```python
from build123d import *

# Parameters (mm, degrees)
BOSS_EXTRUDE1_DEPTH = 20
SKETCH2_R           = 4.835
BOSS_EXTRUDE2_DEPTH = 4
CUT_EXTRUDE1_REACH  = 64.738
SKETCH3_R           = 7.665
CUT_EXTRUDE2_DEPTH  = 10
SKETCH5_W           = 6
SKETCH5_H           = 4
CUT_EXTRUDE3_DEPTH  = 10
CUT_EXTRUDE4_REACH  = 64.738
SKETCH6_R           = 1.165


with BuildPart() as part:
    # Sketch1 → Boss-Extrude1 (new body)
    with BuildSketch(Plane.XY):
        Polygon((-40.25, -10), (-40.25, -6), (-50, -6), (-56, -6), (-56, 6), (-50, 6), (-40.25, 6), (-40.25, 10), (0, 10), (2.25, 10), (2.25, 6), (0, 6), (-9.75, 6), (-9.75, -6), (0, -6), (2.25, -6), (2.25, -10), (0, -10), align=None)
    extrude(amount=BOSS_EXTRUDE1_DEPTH)

    # Sketch2 → Boss-Extrude2 (add)
    with BuildSketch(Plane.XZ.offset(6)):
        with Locations(Location((-50, 10, 0), (0, 0, 180))):
            Circle(SKETCH2_R)
    boss_extrude2 = extrude(amount=BOSS_EXTRUDE2_DEPTH)

    # Cut-Extrude1: up to this face of the body (flat: up to its plane)
    cut_extrude1_end = Plane(part.part.faces().sort_by_distance((-19, 10, 10))[0])
    # Sketch3 → Cut-Extrude1 (cut, up to the picked face)
    with BuildSketch(Plane.XZ.offset(10), mode=Mode.PRIVATE) as cut_extrude1_sk1:
        with Locations((0, 10)):
            Circle(SKETCH3_R)
    cut_extrude1_tool1 = split(extrude(cut_extrude1_sk1.sketch, amount=-CUT_EXTRUDE1_REACH, mode=Mode.PRIVATE), bisect_by=cut_extrude1_end, keep=Keep.BOTH, mode=Mode.PRIVATE)
    add(cut_extrude1_tool1.solids().sort_by(Axis((0, -10, 10), (0, 1, 0)))[0], mode=Mode.SUBTRACT)

    # Mirror1: Boss-Extrude2 across plane
    add(boss_extrude2.mirror(Plane.ZX))

    # Sketch4 → Cut-Extrude2 (cut)
    with BuildSketch(Plane.XY.offset(20)):
        Polygon((-27.5, 2.5), (-22.5, 2.062556682), (-22.5, -2.062556682), (-27.5, -2.5), align=None)
    extrude(amount=-CUT_EXTRUDE2_DEPTH, mode=Mode.SUBTRACT)

    # Sketch5 → Cut-Extrude3 (cut)
    with BuildSketch(Plane.XY.offset(20)):
        with Locations((-30.5, 5.165)):
            Rectangle(SKETCH5_W, SKETCH5_H)
        with Locations((-19.5, 5.165)):
            Rectangle(SKETCH5_W, SKETCH5_H)
        with Locations((-19.5, -5.165)):
            Rectangle(SKETCH5_W, SKETCH5_H)
        with Locations((-30.5, -5.165)):
            Rectangle(SKETCH5_W, SKETCH5_H)
    extrude(amount=-CUT_EXTRUDE3_DEPTH, mode=Mode.SUBTRACT)

    # Cut-Extrude4: up to this face of the body (flat: up to its plane)
    cut_extrude4_end = Plane(part.part.faces().sort_by_distance((-21.952820108, 10, 10))[0])
    # Sketch6 → Cut-Extrude4 (cut, up to the picked face)
    with BuildSketch(Plane.XZ.offset(10), mode=Mode.PRIVATE) as cut_extrude4_sk1:
        with Locations(Location((-30.5, 13, 0), (0, 0, 270))):
            Circle(SKETCH6_R)
    cut_extrude4_tool1 = split(extrude(cut_extrude4_sk1.sketch, amount=-CUT_EXTRUDE4_REACH, mode=Mode.PRIVATE), bisect_by=cut_extrude4_end, keep=Keep.BOTH, mode=Mode.PRIVATE)
    # Sketch6 → Cut-Extrude4 (cut, up to the picked face)
    with BuildSketch(Plane.XZ.offset(10), mode=Mode.PRIVATE) as cut_extrude4_sk2:
        with Locations((-25, 13)):
            Circle(SKETCH6_R)
    cut_extrude4_tool2 = split(extrude(cut_extrude4_sk2.sketch, amount=-CUT_EXTRUDE4_REACH, mode=Mode.PRIVATE), bisect_by=cut_extrude4_end, keep=Keep.BOTH, mode=Mode.PRIVATE)
    # Sketch6 → Cut-Extrude4 (cut, up to the picked face)
    with BuildSketch(Plane.XZ.offset(10), mode=Mode.PRIVATE) as cut_extrude4_sk3:
        with Locations(Location((-19.5, 13, 0), (0, 0, 90))):
            Circle(SKETCH6_R)
    cut_extrude4_tool3 = split(extrude(cut_extrude4_sk3.sketch, amount=-CUT_EXTRUDE4_REACH, mode=Mode.PRIVATE), bisect_by=cut_extrude4_end, keep=Keep.BOTH, mode=Mode.PRIVATE)
    add(cut_extrude4_tool1.solids().sort_by(Axis((-30.5, -10, 13), (0, 1, 0)))[0], mode=Mode.SUBTRACT)
    add(cut_extrude4_tool2.solids().sort_by(Axis((-25, -10, 13), (0, 1, 0)))[0], mode=Mode.SUBTRACT)
    add(cut_extrude4_tool3.solids().sort_by(Axis((-19.5, -10, 13), (0, 1, 0)))[0], mode=Mode.SUBTRACT)


solid = part.part
```
Geometry: final body of the model. Coordinates: model frame, mm. A direction names the side the tool comes from. Give positions to 0.01 mm unless a question says otherwise; leave off trailing zeros. Order: outer loops, then holes, each group sorted by start corner. A loop starts at its lowest first (then second) coordinate and runs counter-clockwise, first axis right, second up. Notation, with made-up numbers: (46.5, 27) -> (67.5, 27) arc R20 cw to (67.5, 32) -> close; hole circle Ø8 at (-27, 52). An arc over 180 degrees is marked (long way). Write each question's results on one line, items separated by ' | '. Start each with the question number.
1) Section A-A (x = 0). Return loops of the section in (y, z) (3 decimals), then the cut area to 3 significant figures.
2) Line query: line 1 (X direction, y = -1.25, z = 13) (3 decimals); line 2 (X direction, y = 4, z = 13) (3 decimals); line 3 (Z direction, x = 0, y = 7.15) (3 decimals). Output: solid intervals per line, ascending. Write a range as from..to.
3) Section D-D (x = -25). Return loops of the section in (y, z) (3 decimals), then the cut area to 3 significant figures.
4) Section B-B (z = 18.25). Count the separate pieces of the cut face and the enclosed holes in it, then the cut area to 3 significant figures.
5) Set-up query: faces 1 (the flat face through (-8, -6, 10)), 2 (the flat face through (-56, 0, 10)), 3 (the cylindrical face through (-45.17, 7.97, 9.79)), 4 (the flat face through (-22.5, 5, 15)). Return all of +Z, -Z, +X, -X, +Y, -Y with unobstructed straight access to the full face (end or side cutting, diameter ignored); none if empty.
6) Section C-C (y = -1.5). Return loops of the section in (x, z) (3 decimals), then the cut area to 3 significant figures.
7) First-contact query: pin 1 (3 mm diameter, centred on x = -5.5, z = 7.5, fed in from -Y); pin 2 (9.5 mm diameter, centred on y = -1, z = 12, fed in from +X); pin 3 (3 mm diameter, centred on y = -9, z = 9, fed in from -X) (3 decimals); pin 4 (1.2 mm diameter, centred on x = -19, y = -5, fed in from +Z). Flat tips, straight axial feed; report the tip coordinate or a pass-through.
8) Draft query along X for faces 5 (the flat face through (-9.75, 0, 10)), 6 (the flat face through (-25.035, 2.284, 15.07)), 7 (the flat face through (-50, 10, 10)), 8 (the flat face through (-20, 3.165, 15)). Return one class per face: pulls with the +X half, pulls with the -X half, needs draft (parallel to the pull), parting line crosses it, or undercut.
Calculated:
1) outline: (-10, 0) -> (-6, 0) -> (-6, 2.335) -> (-10, 2.335) -> close; (-10, 17.665) -> (-6, 17.665) -> (-6, 20) -> (-10, 20) -> close; (6, 0) -> (10, 0) -> (10, 2.335) -> (6, 2.335) -> close; (6, 17.665) -> (10, 17.665) -> (10, 20) -> (6, 20) -> close | area: 37.4 mm2
2) line 1: -56..-31.665, -29.335..-27.5, -22.5..-20.665, -18.335..-9.75 | line 2: -56..-33.5, -27.5..-26.165, -23.835..-22.5, -16.5..-9.75 | line 3: 0..2.335, 17.665..20
3) outline: (-10, 0) -> (10, 0) -> (10, 11.835) -> (2.281, 11.835) -> (2.281, 10) -> (-2.281, 10) -> (-2.281, 11.835) -> (-10, 11.835) -> close; (-10, 14.165) -> (-2.281, 14.165) -> (-2.281, 20) -> (-10, 20) -> close; (2.281, 14.165) -> (10, 14.165) -> (10, 20) -> (2.281, 20) -> close | area: 318 mm2
4) separate pieces: 1 | enclosed holes: 5 | area: 776 mm2
5) face 1: +Z, -Z, +X | face 2: +Z, -Z, -X, +Y, -Y | face 3: +Y | face 4: +Z
6) outline: (-56, 0) -> (-9.75, 0) -> (-9.75, 20) -> (-22.5, 20) -> (-22.5, 10) -> (-27.5, 10) -> (-27.5, 20) -> (-56, 20) -> close; hole circle Ø2.33 at (-30.5, 13); hole circle Ø2.33 at (-19.5, 13) | area: 866 mm2
7) pin 1: through | pin 2: x = -9.75 | pin 3: x = -54.835 | pin 4: z = 10
8) face 5: pulls with the +X half | face 6: undercut | face 7: needs draft | face 8: undercut
